The listing builds one solid part. Answer for the finished solid, in the listing's coordinates (mm). Round coordinates to 2 decimals unless told otherwise and drop trailing zeros. Write each loop counter-clockwise with the first axis right and the second up, starting at its lowest first coordinate (ties: lowest second). Pieces come first, ordered by that corner, then holes. Notation, with made-up numbers: M 44.5,33 L 50.5,33 A36 ccw 50.5,67 Z; hole C 60,61.5 d11. An arc over 180 degrees is marked long. One line per item, written item: value. Start each with the question number.
(1) Consider probe 1 along Y at (x, z) = (-61, 308); probe 2 along Z at (x, y) = (-74.5, 1607); probe 3 along Z at (x, y) = (-55, 1475). Determine where each line is inside the solid, lowest interval first.
(2) Given P1, Ø12, axis at x = -82, y = 260.5, coming from the -Z side; P2, Ø1.5, axis at x = -84.5, y = 1159, coming from the -Z side; P3, Ø1.5, axis at x = 2.5, z = 133.5, coming from the -Y side; P4, Ø4, axis at x = -52.5, z = 636, coming from the -Y side, each flat-ended and moving along its own axis, determine where each tip first touches the part or whether it passes through.
(3) Section D-D (y = 246.5) is taken. Determine the outline of the cut face in (x, z).
(4) Section C-C (z = 457.5) is taken. Determine the outline of the cut face in (x, y), plus the area to 3 significant figures.
(5) Section B-B (x = -92) is taken. Determine the outline of the cut face in (y, z), plus the area to 3 significant figures.
(6) Section A-A (y = 646) is taken. Determine the outline of the cut face in (x, z).
```python
from build123d import *

# Parameters (mm, degrees)
F1_DEPTH  = 120
F2_R      = 15
F3_DEPTH  = 20
F6_DEPTH  = 120
F7_DEPTH  = 29
F8_DEPTH  = 150
F11_R     = 15
F12_DEPTH = 10


# Not quite as in the source:
# - a pattern or mirror of a feature is missing from the dataset's text; its kind, count and spacing are read off the source's solid


with BuildPart() as f1:
    # F0 (on Right) → F1 (new body)
    with BuildSketch(Plane.YZ):
        Polygon((0, 120), (0, 0), (700, 0), (760, 0), (873.1370849898, 113.1370849898), (873.1370849898, 493.1370849898), (1106.4823227814, 726.4823227814), (1556.4823227814, 726.4823227814), (1556.4823227814, 846.4823227814), (1056.7766952966, 846.4823227814), (753.1370849898, 542.8427124746), (753.1370849898, 162.8427124746), (710.2943725152, 120), (700, 120), align=None)
    extrude(amount=-F1_DEPTH)

    # F2 (on face) → F3 (join)
    with BuildSketch(Plane.XY.offset(120)):
        with BuildLine():
            Line((0, 0), (-120, 0))
            ThreePointArc((-120, 0), (-60, -60), (0, 0))
        make_face()
        with Locations((-60, -30)):
            Circle(F2_R, mode=Mode.SUBTRACT)
    f3 = extrude(amount=-F3_DEPTH)

    # F3_copies: F3 across plane
    add(f3.mirror(Plane(origin=(0, 0, 60), x_dir=(-1, 0, 0), z_dir=(0, 0, -1))))

    # F5 (on face) → F6 (join)
    with BuildSketch(Plane.XY.offset(846.4823227814)):
        Polygon((-120, 1556.4823227814), (-60, 1556.4823227814), (0, 1556.4823227814), (0, 1666.4823227814), (-120, 1666.4823227814), align=None)
        with BuildLine():
            ThreePointArc((-7.5, 1611.4823227814), (-22.8768939877, 1574.3592167691), (-60, 1558.9823227814))
            ThreePointArc((-60, 1558.9823227814), (-97.1231060123, 1648.6054287937), (-7.5, 1611.4823227814))
        make_face(mode=Mode.SUBTRACT)
        with BuildLine():
            ThreePointArc((-7.5, 1611.4823227814), (-97.1231060123, 1648.6054287937), (-60, 1558.9823227814))
            ThreePointArc((-60, 1558.9823227814), (-22.8768939877, 1574.3592167691), (-7.5, 1611.4823227814))
        make_face()
        with BuildLine():
            Line((-120, 1666.4823227814), (0, 1666.4823227814))
            ThreePointArc((0, 1666.4823227814), (-60, 1703.8881069987), (-120, 1666.4823227814))
        make_face()
    extrude(amount=-F6_DEPTH)

    # F5 (on face) → F7 (join)
    with BuildSketch(Plane.XY.offset(846.4823227814)):
        with BuildLine():
            ThreePointArc((-7.5, 1611.4823227814), (-97.1231060123, 1648.6054287937), (-60, 1558.9823227814))
            ThreePointArc((-60, 1558.9823227814), (-22.8768939877, 1574.3592167691), (-7.5, 1611.4823227814))
        make_face()
    extrude(amount=F7_DEPTH)

    # F5 (on face) → F8 (join)
    with BuildSketch(Plane.XY.offset(846.4823227814)):
        with BuildLine():
            ThreePointArc((-7.5, 1611.4823227814), (-97.1231060123, 1648.6054287937), (-60, 1558.9823227814))
            ThreePointArc((-60, 1558.9823227814), (-22.8768939877, 1574.3592167691), (-7.5, 1611.4823227814))
        make_face()
    extrude(amount=-F8_DEPTH)

    # F11 (on offset) → F12 (join)
    with BuildSketch(Plane.XY.offset(115)):
        with BuildLine():
            Line((89.2130512357, 626.3729619547), (-2.970210975, 665.1317824757))
            Line((-2.970210975, 665.1317824757), (-2.970210975, 549.5901644294))
            Line((-2.970210975, 549.5901644294), (89.2130512357, 588.3489849504))
            ThreePointArc((89.2130512357, 588.3489849504), (101.8435068324, 607.3609734525), (89.2130512357, 626.3729619547))
        make_face()
        with Locations((79.0183379768, 607.3609734525)):
            Circle(F11_R, mode=Mode.SUBTRACT)
    f12 = extrude(amount=-F12_DEPTH)

    # F12_copies: F12 across plane
    add(f12.mirror(Plane(origin=(0, 0, 80), x_dir=(-1, 0, 0), z_dir=(0, 0, -1))))


solid = f1.part
```
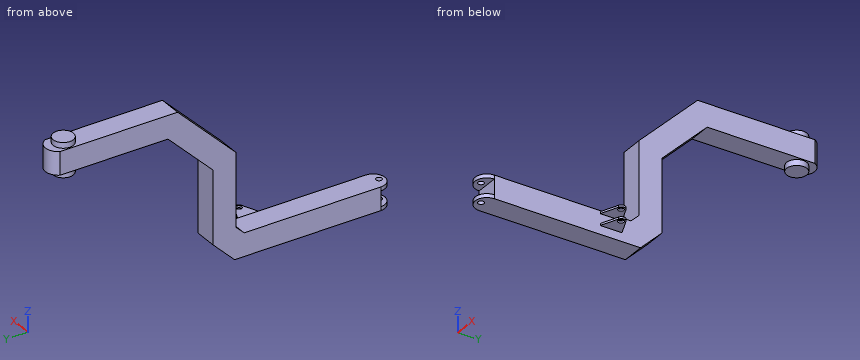
Recorded:
1. probe 1: y = 753.14 to 873.14
1. probe 2: z = 696.48 to 875.48
1. probe 3: z = 726.48 to 846.48
2. P1: stops at z = 0
2. P2: stops at z = 726.48
2. P3: passes through
2. P4: stops at y = 844.29
3. outline: M -120,0 L 0,0 L 0,120 L -120,120 Z
4. outline: M -120,753.14 L 0,753.14 L 0,873.14 L -120,873.14 Z
4. area: 14,400 mm2
5. outline: M -50.75,0 L 760,0 L 873.14,113.14 L 873.14,493.14 L 1106.48,726.48 L 1569.86,726.48 L 1569.86,696.48 L 1653.1,696.48 L 1653.1,726.48 L 1695.73,726.48 L 1695.73,846.48 L 1653.1,846.48 L 1653.1,875.48 L 1569.86,875.48 L 1569.86,846.48 L 1056.78,846.48 L 753.14,542.84 L 753.14,162.84 L 710.29,120 L -50.75,120 L -50.75,100 L 0,100 L 0,20 L -50.75,20 Z
5. area: 273,000 mm2
6. outline: M -120,0 L 0,0 L 0,45 L 42.53,45 L 42.53,55 L 0,55 L 0,105 L 42.53,105 L 42.53,115 L 0,115 L 0,120 L -120,120 Z
